Job drawing, mm, ordinate dimensions from the low corner. One solid piece. A direction names the side the tool comes from. Give positions to 0.01 mm unless a question says otherwise; leave off trailing zeros. Write each loop counter-clockwise with the first axis right and the second up, starting at its lowest first coordinate (ties: lowest second). Pieces come first, ordered by that corner, then holes. Notation, with made-up numbers: (4, -13) - (60, -13) arc R23 cw to (60, 21) - close; hole circle Ø8 at (-38.5, 16.25). An arc over 180 degrees is marked (long way). Answer as a JSON object with one key per item and string values.
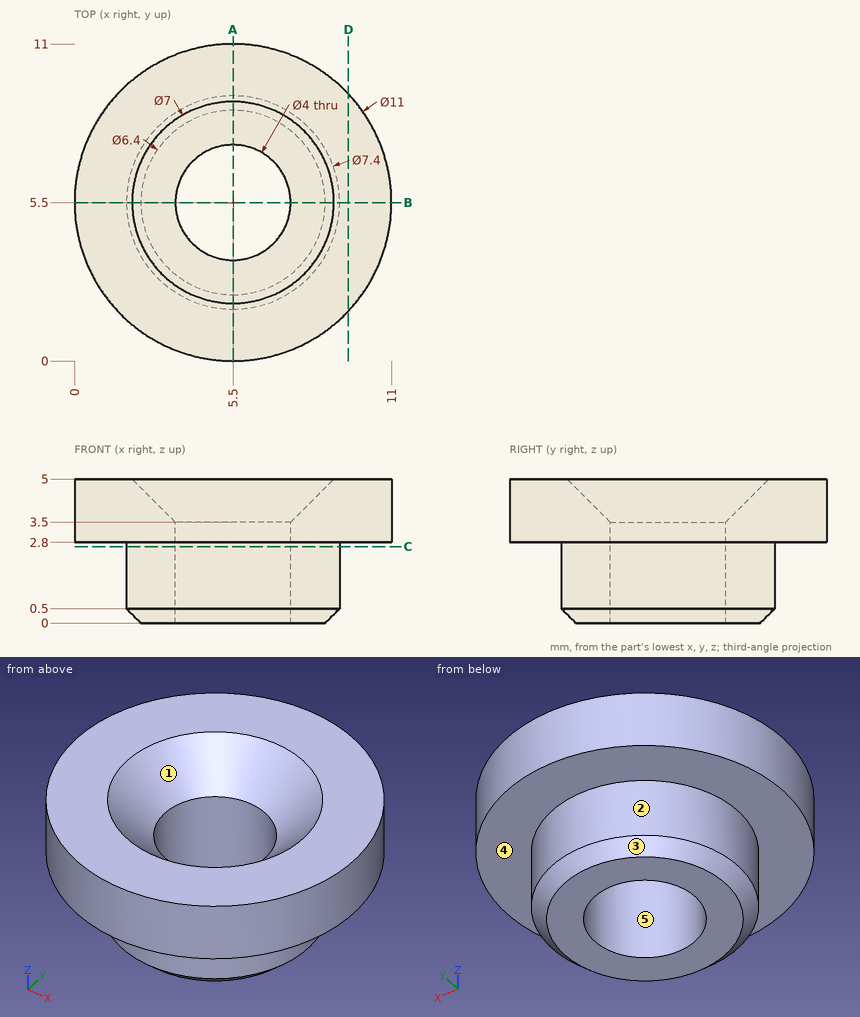
Item 1: Mould opens along Y. For the marked faces 3, 4 and 5 say: +Y half, -Y half, draft (parallel to the pull), parting line (faces both ways), or undercut.
Entries:
{"face 3": "parting line", "face 4": "draft", "face 5": "undercut"}
Item 2: Cut at A-A (x = 5.5). Give the cut face in (y, z).
Entries:
{"outline": "(0, 2.8) - (1.8, 2.8) - (1.8, 0.5) - (2.3, 0) - (3.5, 0) - (3.5, 3.5) - (2, 5) - (0, 5) - close; (7.5, 0) - (8.7, 0) - (9.2, 0.5) - (9.2, 2.8) - (11, 2.8) - (11, 5) - (9, 5) - (7.5, 3.5) - close"}
Item 3: Cut at C-C (z = 2.65). Give the cut face in (x, y).
Entries:
{"outline": "circle Ø7.4 at (5.5, 5.5); hole circle Ø4 at (5.5, 5.5)"}
Item 4: Probe line 1 (X direction, y = 5.5, z = 0.9); line 2 (Z direction, x = 10, y = 7.25); line 3 (Y direction, x = 5, z = 4.6). List the from-to ranges inside material, lowest first. Write a range as from..to.
Entries:
{"line 1": "1.8..3.5, 7.5..9.2", "line 2": "2.8..5", "line 3": "0.02..2.44, 8.56..10.98"}
Item 5: Flat gauge pins, fed straight in: P1, Ø1, axis at y = 1.5, z = 2.5, coming from the -X side; P2, Ø1, axis at x = 4.5, z = 1.5, coming from the +Y side; P3, Ø4.5, axis at x = 5.5, y = 5.5, coming from the +Z side; P4, Ø3, axis at y = 4, z = 3.5, coming from the +X side. Where does each tip first touch, or does it go through?
Entries:
{"P1": "x = 1.34", "P2": "y = 9.17", "P3": "z = 3.75", "P4": "x = 11"}
Item 6: Cut at D-D (x = 9.5). Give the cut face in (y, z), and give its area (3 significant figures).
Entries:
{"outline": "(1.73, 2.8) - (9.27, 2.8) - (9.27, 5) - (1.73, 5) - close", "area": "16.6 mm2"}
Item 7: Which spindle directions (+Z, -Z, +X, -X, +Y, -Y) get a long thin tool onto all of the face, cutting with end or side? Do the marked faces 1 and 2. Say none if no direction does.
Entries:
{"face 1": "+Z", "face 2": "-Z"}
